Verification items for this drawing (mm, ordinates from the low corner). A direction names the side the tool comes from. Coordinates: 2 decimals unless noted, no trailing zeros. Order: outer loops, then holes, each group sorted by start corner. A loop starts at its lowest first (then second) coordinate and runs counter-clockwise, first axis right, second up. Notation, with made-up numbers: M 88,-2.75 L 124,-2.75 A21 ccw 124,20.25 Z; hole C 35.5,-4 d2. An arc over 180 degrees is marked long. One line per item, written item: value. Start each with the question number.
1) Sectioned sample at C-C, the plane y = 17. Enter the section's corners in (x, z).
2) Draft check along Y on the marked faces 1, 2 and 3. Enter one of: pulls with the +Y half, pulls with the -Y half, needs draft (parallel to the pull), parting line crosses it, or undercut.
3) Thickness scan on L1, parallel to Y at x = 25.4, z = 5.25; L2, parallel to Z at x = 25.4, y = 30.75; L3, parallel to Z at x = 3, y = 16. Record the ranges inside material, lowest first. Write a range as from..to.
4) Sectioned sample at D-D, the plane y = 32. Enter the section's corners in (x, z).
5) Access from +Z, -Z, +X, -X, +Y, -Y to the whole of each face (thin tool, end or side, straight path). Record for the marked faces 4 and 5.
6) Sectioned sample at B-B, the plane x = 25.4. State how many separate pieces and enclosed holes the cut face has.
7) Go/stop test with flat-tipped pins: P1, Ø1.5, axis at y = 8.5, z = 4.5, coming from the -X side (1 decimal); P2, Ø2.5, axis at x = 25.4, y = 25.4, coming from the +Z side; P3, Ø4, axis at x = 25.4, y = 25.4, coming from the -Z side; P4, Ø3, axis at x = 26.5, z = 3, coming from the -Y side (1 decimal). Record where each tip stops, or that it passes through.
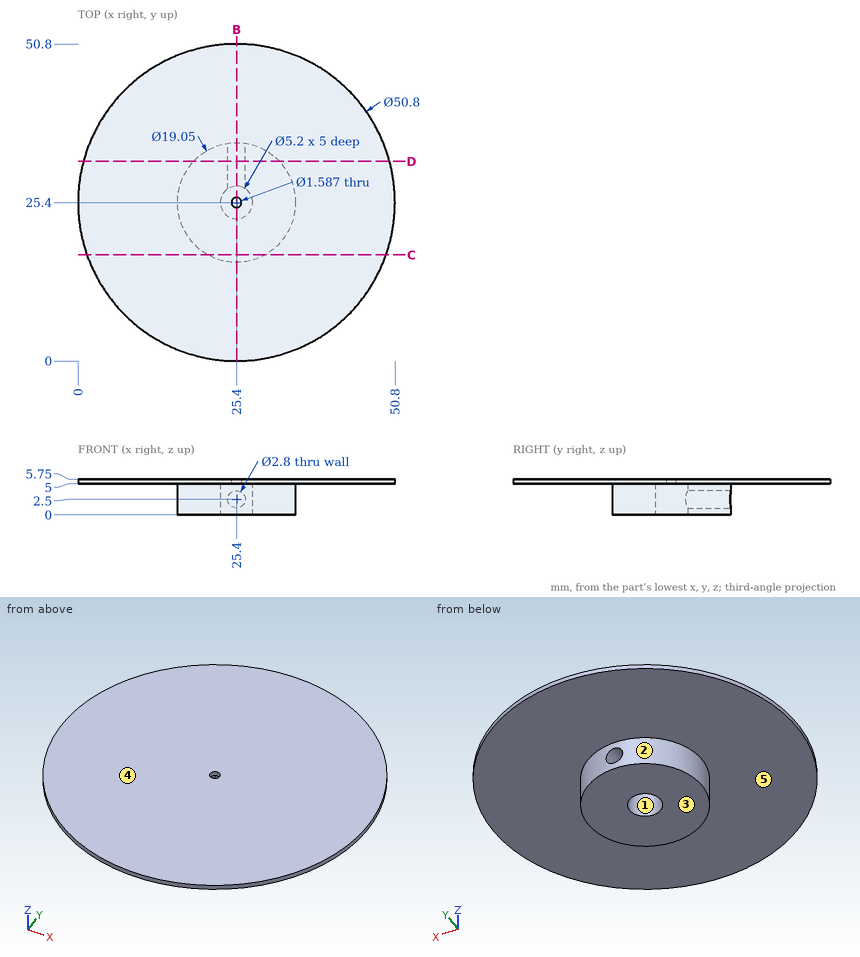
Final values:
1. outline: M 1.43,5 L 20.91,5 L 20.91,0 L 29.89,0 L 29.89,5 L 49.37,5 L 49.37,5.75 L 1.43,5.75 Z
2. face 1: undercut
2. face 2: parting line crosses it
2. face 3: needs draft
3. L1: y = 0..24.61, 26.19..50.8
3. L2: z = 0..1.1, 3.9..5.75
3. L3: z = 5..5.75
4. outline: M 0.87,5 L 18.53,5 L 18.53,0 L 32.27,0 L 32.27,5 L 49.93,5 L 49.93,5.75 L 0.87,5.75 Z; hole C 25.4,2.5 d2.8
5. face 4: +Z, +X, -X, +Y, -Y
5. face 5: -Z
6. separate pieces: 3
6. enclosed holes: 0
7. P1: stops at x = 6
7. P2: stops at z = 5.75
7. P3: stops at z = 5
7. P4: stops at y = 15.9
